Design review of the part built by this model. Coordinates are the model's own, in mm. Face numbers are marked on the shaded views. A direction names the side the tool comes from. Round coordinates to 2 decimals unless told otherwise and drop trailing zeros. Order: outer loops, then holes, each group sorted by start corner. A loop starts at its lowest first (then second) coordinate and runs counter-clockwise, first axis right, second up. Notation, with made-up numbers: M 38.5,11 L 73.5,11 A19 ccw 73.5,34 Z; hole C -15,51.25 d11. An arc over 180 degrees is marked long. Write each question's results on one line, items separated by ' | '. Start each with the question number.
Item 1: Machinability: for the marked faces 1 and 2, which of the approach directions +Z, -Z, +X, -X, +Y, -Y give a long, thin tool a straight path to every point of the face, cutting with its end or side? Answer none if there is none.
Item 2: Take a section at C-C, the plane x = -0.25. Write out the cut boundary in (y, z).
Item 3: Take a section at D-D, the plane y = -1.9. Write out the cut boundary in (x, z) (3 decimals), plus the area to 3 significant figures.
Item 4: Clearance check with a flat-ended pin moving along its axis: pin 1 (2.5 mm diameter, centred on x = 0, y = 1, fed in from +Z). State where the tip first meets the part, or that it passes through.
Item 5: The part is to be moulded in two halves that separate along X. For the marked faces 3, 4 and 5, say which applies: +X half, -X half, draft (parallel to the pull), parting line (faces both ways), or undercut.
Item 6: Take a section at B-B, the plane z = -0.3. Write out the cut boundary in (x, y), plus the area to 3 significant figures.
Item 7: Wall thickness on line 1 (Y direction, x = 1.5, z = 1.1); line 2 (Z direction, x = -1, y = -1.4); line 3 (X direction, y = -2.15, z = 1.45) (3 decimals): over which ranges is each line inside the solid? List them lowest first. Write a range as [from, to].
Item 8: Take a section at A-A, the plane y = 1.27. Write out the cut boundary in (x, z) (3 decimals).
Autodesk Inventor part; units mm, degrees
ref_plane "YZ Plane" through (0, 0, 0) normal (1, 0, 0) x (0, 1, 0)
ref_plane "XZ Plane" through (0, 0, 0) normal (0, 1, 0) x (-1, 0, 0)
ref_plane "XY Plane" through (0, 0, 0) normal (0, 0, 1) x (1, 0, 0)
sketch "Sketch1" plane through (0, 0, 0) normal (0, 0, 1) x (1, 0, 0)
  line L0 (-3.275, -2.95) -> (3.275, -2.95)
  line L1 (3.275, -2.95) -> (3.275, 2.95)
  line L2 (3.275, 2.95) -> (-3.275, 2.95)
  line L3 (-3.275, 2.95) -> (-3.275, -2.95)
  line L4 (-3.275, -2.95) -> (3.275, 2.95) construction
  line L5 (3.275, -2.95) -> (-3.275, 2.95) construction
  point P0 (0, 0)
  dimension "d0" = 6.55
  dimension "d1" = 5.9
extrude "Extrusion1" add sketch "Sketch1" along normal blind 2
sketch "Sketch2" plane through (0, 0, 2) normal (0, 0, 1) x (1, 0, 0)
  line L0 (-3.275, -2.95) -> (3.275, -2.95)
  line L1 (3.275, -2.95) -> (3.275, 2.95)
  line L2 (3.275, 2.95) -> (-3.275, 2.95)
  line L3 (-3.275, 2.95) -> (-3.275, -2.95)
  line L4 (-2.775, 2.45) -> (2.775, 2.45)
  line L5 (2.775, 2.45) -> (2.775, -2.45)
  line L6 (2.775, -2.45) -> (-2.775, -2.45)
  line L7 (-2.775, -2.45) -> (-2.775, 2.45)
  point P0 (0, 0)
  dimension "d4" = 0.5
extrude "Extrusion2" cut sketch "Sketch2" against normal blind 1 contours L4 L5 L6 L7
sketch "Sketch3" plane through (0, 0, 1) normal (0, 0, 1) x (1, 0, 0)
  line L0 (-2.775, 2.45) -> (2.775, 2.45)
  line L1 (-2.775, -2.45) -> (-2.775, 2.45)
  line L2 (2.775, -2.45) -> (-2.775, -2.45)
  line L3 (2.775, 2.45) -> (2.775, -2.45)
  line L4 (-1.17, 1.5) -> (1.83, 1.5)
  line L5 (1.83, 1.5) -> (1.83, -1.5)
  line L6 (1.83, -1.5) -> (-1.17, -1.5)
  line L7 (-1.17, -1.5) -> (-1.17, 1.5)
  line L8 (-1.17, 1.5) -> (1.83, -1.5) construction
  line L9 (1.83, 1.5) -> (-1.17, -1.5) construction
  line L10 (-2.775, 2.45) -> (-1.775, 2.45)
  line L11 (-1.775, 2.45) -> (-1.775, -2.45)
  line L12 (-1.775, -2.45) -> (-2.775, -2.45)
  line L13 (-2.775, -2.45) -> (-2.775, 2.45)
  point P0 (0, 0)
  point P1 (0.33, 0)
  dimension "d7" = 3
  dimension "d8" = 3
  dimension "d9" = 0.33
  dimension "d10" = 0
  dimension "d11" = 1
  dimension "d13" = 0
  dimension "d14" = 0
  dimension "d15" = 0
extrude "Extrusion3" add sketch "Sketch3" along normal blind 0.55 contours L0 L11 L2 L1 | L4 L5 L6 L7
sketch "Sketch4" plane through (0, 0, 0) normal (0, 0, -1) x (-1, 0, 0)
  line L0 (3.275, -2.95) -> (-3.275, -2.95)
  line L1 (3.275, 2.95) -> (3.275, -2.95)
  line L2 (-3.275, 2.95) -> (3.275, 2.95)
  line L3 (-3.275, -2.95) -> (-3.275, 2.95)
  circle A0 centre (2, 1.27) radius 0.23
  circle A1 centre (2, -1.27) radius 0.23
  line L4 (1.775, 2.45) -> (1.775, -2.45)
  line L5 (2, 1.27) -> (2, -1.27)
  line L6 (0, 0) -> (3.275, 0)
  point P0 (2, 0)
  dimension "d18" = 2
  dimension "d19" = 2
  dimension "d20" = 2.54
  dimension "d21" = 0.46
  dimension "d22" = 0.46
extrude "Extrusion4" add sketch "Sketch4" along normal blind 2 contours A0 L4 | A1 L4 | A0 L4 | L4 A1
equation "\"d0\" = MPPCHeight"
equation "\"d1\" = MPPCWidth"
equation "\"d19\" = d18"
equation "\"d22\" = d21"
equation "\"MPPCWidth\" = 5.9"
equation "\"MPPCHeight\" = 6.55"
properties part number "MPPC" material "ABS Plastic"
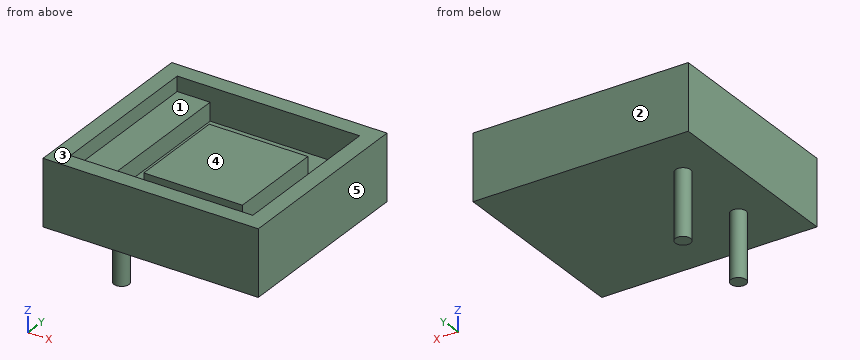
Results list:
1) face 1: +Z | face 2: +Z, -Z, +X, -X, +Y
2) outline: M -2.95,0 L 2.95,0 L 2.95,2 L 2.45,2 L 2.45,1 L 1.5,1 L 1.5,1.55 L -1.5,1.55 L -1.5,1 L -2.45,1 L -2.45,2 L -2.95,2 Z
3) outline: M -3.275,0 L 3.275,0 L 3.275,2 L 2.775,2 L 2.775,1 L -1.775,1 L -1.775,1.55 L -2.775,1.55 L -2.775,2 L -3.275,2 Z | area: 8.10 mm²
4) pin 1: z = 1.55
5) face 3: draft | face 4: undercut | face 5: +X half
6) outline: C -2,-1.27 d0.46; C -2,1.27 d0.46 | area: 0.332 mm²
7) line 1: [-2.95, -2.45], [-1.5, 1.5], [2.45, 2.95] | line 2: [0, 1.55] | line 3: [-3.275, -1.775], [2.775, 3.275]
8) outline: M -3.275,0 L -2.23,0 L -2.23,-2 L -1.77,-2 L -1.77,0 L 3.275,0 L 3.275,2 L 2.775,2 L 2.775,1 L 1.83,1 L 1.83,1.55 L -1.17,1.55 L -1.17,1 L -1.775,1 L -1.775,1.55 L -2.775,1.55 L -2.775,2 L -3.275,2 Z
